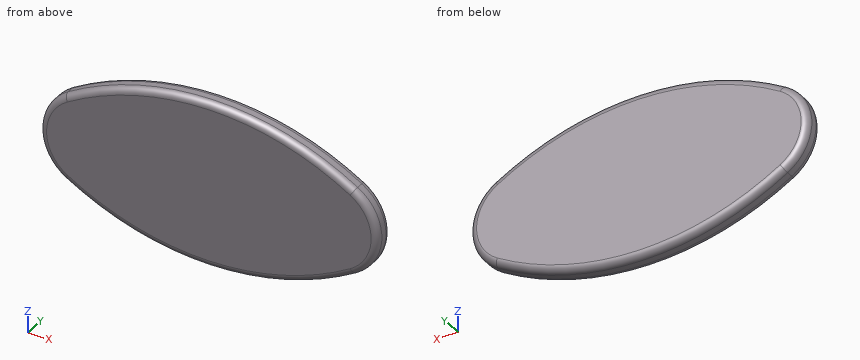
```python
from build123d import *

# Parameters (mm, degrees)
F1_DEPTH = 30
F2_R     = 10


with BuildPart() as f1:
    # F0 (on Front) → F1 (new body)
    with BuildSketch(Plane.XZ):
        with BuildLine():
            ThreePointArc((218.587182, 64.311969), (0, 124.857114), (-218.587182, 64.311969))
            ThreePointArc((-218.587182, 64.311969), (-255, 0), (-218.587182, -64.311969))
            ThreePointArc((-218.587182, -64.311969), (0, -124.857114), (218.587182, -64.311969))
            ThreePointArc((218.587182, -64.311969), (255, 0), (218.587182, 64.311969))
        make_face()
    extrude(amount=F1_DEPTH)

    # F2
    f2_edges = [f1.edges().sort_by_distance(p)[0] for p in [
        (0, -30, -124.857114),
        (0, 0, -124.857114),
    ]]
    fillet(f2_edges, radius=F2_R)


solid = f1.part
```
The listing builds one solid part. Answer for the finished solid, in the listing's coordinates (mm). Give positions to 0.01 mm unless a question says otherwise; leave off trailing zeros. Loops run counter-clockwise (first coordinate to the right, second up) from the corner with the lowest first, then second, coordinate; pieces in that order, holes last. Notation, with made-up numbers: M 67,-21 L 117,-21 A19 cw 117,8 Z; hole C 50,66.5 d4. An arc over 180 degrees is marked long. One line per item, written item: value.
Q1. Find the intervals of material crossed by line 1 (Z direction, x = 81.5, y = -20); line 2 (Z direction, x = -133.5, y = -9.75); line 3 (X direction, y = -15.75, z = -93), in increasing order. Write a range as from..to.
Working result:
line 1: z = -116.97..116.97
line 2: z = -103.33..103.33
line 3: x = -161.41..161.41
Q2. Flat-ended cylindrical pins translate along their axes: P1, Ø1, axis at y = -17.5, z = 13.5, coming from the -X side; P2, Ø1.5, axis at y = -10.5, z = -53.5, coming from the +X side; P3, Ø1, axis at x = -61, y = -3, coming from the -Z side. Find the tip coordinate at first contact, or state that the pin passes through.
Working result:
P1: stops at x = -253.86
P2: stops at x = 233.31
P3: stops at z = -118.04
Q3. A cutting plane is placed at A-A on y = -4.75. Determine the outline of the cut face in (x, z), then the cut area to 3 significant figures.
Working result:
outline: M -217.82,-63.04 A423.37 ccw 217.82,-63.04 A73.51 ccw 217.82,63.04 A423.37 ccw -217.82,63.04 A73.51 ccw Z
area: 96,900 mm^2
